Autodesk Inventor part; units mm, degrees
ref_plane "YZ Plane" through (0, 0, 0) normal (1, 0, 0) x (0, 1, 0)
ref_plane "XZ Plane" through (0, 0, 0) normal (0, 1, 0) x (-1, 0, 0)
ref_plane "XY Plane" through (0, 0, 0) normal (0, 0, 1) x (1, 0, 0)
sketch "Sketch1" plane through (0, 0, 0) normal (0, 1, 0) x (-1, 0, 0)
  line L0 (3, 10) -> (-3, 10)
  line L1 (-3, 10) -> (-3, -10)
  line L2 (-3, -10) -> (3, -10)
  line L3 (3, -10) -> (3, 10)
  line L4 (3, 10) -> (-3, -10) construction
  line L5 (-3, 10) -> (3, -10) construction
  circle A0 centre (0, 10) radius 3
  circle A1 centre (0, -10) radius 3
  line L6 (-3, -10) -> (-7, -10)
  line L7 (-7, -10) -> (-7, -6)
  line L8 (-7, -6) -> (-7, -4)
  line L9 (-7, -4) -> (-3, -4)
  line L10 (-7, -4) -> (-7, -7)
  circle A2 centre (-7, -7) radius 3
  line L11 (-3, -4) -> (-3, -10)
  point P0 (0, 0)
  dimension "d0" = 6
  dimension "d1" = 20
  dimension "d2" = 6
  dimension "d4" = 6
  dimension "d5" = 4
  dimension "d6" = 4
  dimension "d7" = 2
  dimension "d10" = 3
  dimension "d11" = 6
extrude "Extrusion1" add sketch "Sketch1" along normal blind 1.5 contours A0 L0 | L0 A0 | L3 A1 L1 A0 | A1 L2 | L2 A1 | A2 L7 L8 | L8 L7 A2
sketch "Sketch2" plane through (0, 1.5, 0) normal (0, 1, 0) x (1, 0, 0)
  line L0 (3, -10) -> (3, 10)
  arc A0 (3, 10) -> (-3, 10) centre (0, 10) ccw
  line L1 (-3, 10) -> (-3, -10)
  arc A1 (-3, -10) -> (3, -10) centre (0, -10) ccw
  circle A2 centre (0, 10) radius 1.5
  circle A3 centre (0, -10) radius 1.5
  line L2 (3, 10) -> (7, 10)
  line L3 (7, 10) -> (7, 4)
  line L4 (7, 4) -> (3, 4)
  line L5 (3, 4) -> (3, 10)
  point P0 (0, 0)
  dimension "d14" = 3
  dimension "d15" = 3
  dimension "d16" = 4
  dimension "d17" = 6
extrude "Extrusion2" cut sketch "Sketch2" against normal blind 1.5 contours L0 L2 L3 L4 | A2 | A3
sketch "Sketch3" plane through (0, 1.5, 0) normal (0, 1, 0) x (1, 0, 0)
  line L0 (3, -10) -> (3, 10)
  arc A0 (3, 10) -> (-3, 10) centre (0, 10) ccw
  line L1 (-3, 10) -> (-3, -10)
  line L2 (3, 10) -> (7, 10)
  line L3 (7, 10) -> (7, 4)
  line L4 (7, 4) -> (3, 4)
  line L5 (3, 4) -> (3, 10)
  point P0 (0, 0)
  dimension "d20" = 4
  dimension "d21" = 6
  dimension "d22" = 4
extrude "Extrusion3" add sketch "Sketch3" against normal blind 1.5
sketch "Sketch4" plane through (0, 1.5, 0) normal (0, 1, 0) x (1, 0, 0)
  arc A0 (7, 4) -> (7, 10) centre (7, 7) ccw
  circle A1 centre (7, 7) radius 1.5
  point P0 (0, 0)
  dimension "d25" = 3
extrude "Extrusion4" cut sketch "Sketch4" against normal blind 1.5
sketch "Sketch5" plane through (0, 0, 0) normal (0, -1, 0) x (1, 0, 0)
  circle A0 centre (7, -7) radius 1.5
  circle A1 centre (0, 10) radius 1.5
  circle A2 centre (0, -10) radius 1.5
  arc A3 (7, -10) -> (7, -4) centre (7, -7) ccw
  arc A4 (3, 10) -> (-3, 10) centre (0, 10) ccw
  arc A5 (-3, -10) -> (3, -10) centre (0, -10) ccw
  circle A6 centre (0, 10) radius 0.1
  circle A7 centre (0, -10) radius 0.1
  circle A8 centre (7, -7) radius 0.1
  point P0 (0, 0)
  dimension "d28" = 0.2
  dimension "d29" = 0.2
  dimension "d30" = 0.2
extrude "Extrusion5" add sketch "Sketch5" against normal blind 1.5
properties part number "tahlo3_sablona_20"
Geometry: final body of the model. Coordinates: model frame, mm. A direction names the side the tool comes from. Give positions to 0.01 mm unless a question says otherwise; leave off trailing zeros. Write each loop counter-clockwise with the first axis right and the second up, starting at its lowest first coordinate (ties: lowest second). Pieces come first, ordered by that corner, then holes. Notation, with made-up numbers: (16.25, 87.25) -> (60.25, 87.25) arc R18 ccw to (60.25, 93.25) -> close; hole circle Ø10 at (5, 36). An arc over 180 degrees is marked (long way). Answer as a JSON object with one key per item and string values.
1. Cut plane A-A on y = 0.7. Output: boundary loops of the cut face in (x, z), and give its area (3 significant figures).
Ans:
{"outline": "(-3, -10) arc R3 ccw to (3, -10) -> (7, -10) arc R3 ccw to (7, -4) -> (3, -4) -> (3, 10) arc R3 ccw to (-3, 10) -> close; hole circle Ø0.2 at (0, -10); hole circle Ø0.2 at (0, 10); hole circle Ø0.2 at (7, -7)", "area": "186 mm^2"}
2. Access query for faces 1 (the flat face through (3, 1, 3)), 2 (the flat face through (1, 0, -3)), 3 (the flat face through (5, 1, -10)). Directions: +Z, -Z, +X, -X, +Y, -Y. A direction counts if a zero-diameter tool reaches every point of the face in a straight line with its end or side. Return the directions, or none.
Ans:
{"face 1": "+Z, +X, +Y, -Y", "face 2": "+Z, -Z, +X, -X, -Y", "face 3": "-Z, +X, +Y, -Y"}
3. Cut plane C-C on z = -3. Output: boundary loops of the cut face in (x, y), and give its area (3 significant figures).
Ans:
{"outline": "(-3, 0) -> (3, 0) -> (3, 1.5) -> (-3, 1.5) -> close", "area": "9.00 mm^2"}
4. Contact query for a flat-ended pin moving along its axis: pin 1 (0.8 mm diameter, centred on y = 1, z = 2.5, fed in from +X). Output: stop coordinate, or through.
Ans:
{"pin 1": "stops at x = 3"}
5. Cut plane B-B on x = 5.75. Output: boundary loops of the cut face in (y, z).
Ans:
{"outline": "(0, -10) -> (1.5, -10) -> (1.5, -4) -> (0, -4) -> close"}
6. Ray query, probe 1 along Z at (x, y) = (0, 1.15); probe 2 along X at (y, z) = (0.95, -7); probe 3 along X at (y, z) = (0.9, 10). Return the intervals inside material, ascending. Write a range as from..to.
Ans:
{"probe 1": "z = -13..-10.1, -9.9..9.9, 10.1..13", "probe 2": "x = -3..6.9, 7.1..10", "probe 3": "x = -3..-0.1, 0.1..3"}
